```python
from build123d import *

# Parameters (mm, degrees)
ESBO_O1_W                = 50
ESBO_O1_H                = 11
RESSALTO_EXTRUS_O1_DEPTH = 22.5
ESBO_O2_W                = 46
ESBO_O2_H                = 7
CORTE_EXTRUS_O1_DEPTH    = 20.5
ESBO_O3_W                = 10.97916057
ESBO_O3_H                = 2
CORTE_EXTRUS_O2_DEPTH    = 4
CORTE_EXTRUS_O3_DEPTH    = 4
ESBO_O9_W                = 50
ESBO_O9_H                = 4
RESSALTO_EXTRUS_O4_DEPTH = 7
ESBO_O13_R               = 1.5
CORTE_EXTRUS_O4_DEPTH    = 7
ESBO_O19_W               = 9
ESBO_O19_H               = 4
RESSALTO_EXTRUS_O5_DEPTH = 22.5
ESBO_O20_R               = 1.7
RESSALTO_EXTRUS_O7_DEPTH = 3.5
ESBO_O21_W               = 68.510383691
ESBO_O21_H               = 66.833312069
CORTE_EXTRUS_O7_DEPTH    = 50.144843501
CORTE_EXTRUS_O8_DEPTH    = 35.762993058
RESSALTO_EXTRUS_O9_DEPTH = 3.5
ESBO_O24_R               = 1.6
CORTE_EXTRUS_O9_DEPTH    = 3.5


with BuildPart() as part:
    # Esboço1 → Ressalto-extrusão1 (new body)
    with BuildSketch(Plane(origin=(0, 0, 0), x_dir=(1, 0, 0), z_dir=(0, 1, 0))):
        Rectangle(ESBO_O1_W, ESBO_O1_H)
    extrude(amount=RESSALTO_EXTRUS_O1_DEPTH)

    # Esboço2 → Corte-extrusão1 (cut)
    with BuildSketch(Plane(origin=(0, 22.5, 0), x_dir=(1, 0, 0), z_dir=(0, 1, 0))):
        Rectangle(ESBO_O2_W, ESBO_O2_H)
    extrude(amount=-CORTE_EXTRUS_O1_DEPTH, mode=Mode.SUBTRACT)

    # Esboço3 → Corte-extrusão2 (cut)
    with BuildSketch(Plane(origin=(0, 22.5, 0), x_dir=(1, 0, 0), z_dir=(0, 1, 0))):
        with Locations((0, 4.5)):
            Rectangle(ESBO_O3_W, ESBO_O3_H)
    extrude(amount=-CORTE_EXTRUS_O2_DEPTH, mode=Mode.SUBTRACT)

    # Esboço5 → Corte-extrusão3 (cut)
    with BuildSketch(Plane.XY.offset(5.5)):
        with BuildLine():
            Line((-21, 22.5), (-4.5, 22.5))
            Line((-4.5, 22.5), (-4.5, 11.75))
            ThreePointArc((-4.5, 11.75), (-12.75, 3.5), (-21, 11.75))
            Line((-21, 11.75), (-21, 22.5))
        make_face()
        with BuildLine():
            Line((4.5, 22.5), (21, 22.5))
            Line((21, 22.5), (21, 11.75))
            ThreePointArc((21, 11.75), (12.75, 3.5), (4.5, 11.75))
            Line((4.5, 11.75), (4.5, 22.5))
        make_face()
    extrude(amount=-CORTE_EXTRUS_O3_DEPTH, mode=Mode.SUBTRACT)

    # Esboço9 → Ressalto-extrusão4 (add)
    with BuildSketch(Plane(origin=(0, 0, -5.5), x_dir=(-1, 0, 0), z_dir=(0, 0, -1))):
        with Locations((0, 2)):
            Rectangle(ESBO_O9_W, ESBO_O9_H)
    extrude(amount=RESSALTO_EXTRUS_O4_DEPTH)

    # Esboço13 → Corte-extrusão4 (cut)
    with BuildSketch(Plane(origin=(0, 4, 0), x_dir=(1, 0, 0), z_dir=(0, 1, 0))):
        with Locations(Location((10, 9, 0), (0, 0, 270))):
            Circle(ESBO_O13_R)
        with Locations(Location((5, 9, 0), (0, 0, 270))):
            Circle(ESBO_O13_R)
        with Locations(Location((20, 9, 0), (0, 0, 270))):
            Circle(ESBO_O13_R)
        with Locations(Location((15, 9, 0), (0, 0, 270))):
            Circle(ESBO_O13_R)
        with Locations(Location((0, 9, 0), (0, 0, 270))):
            Circle(ESBO_O13_R)
        with Locations(Location((-5, 9, 0), (0, 0, 270))):
            Circle(ESBO_O13_R)
        with Locations(Location((-10, 9, 0), (0, 0, 270))):
            Circle(ESBO_O13_R)
        with Locations(Location((-15, 9, 0), (0, 0, 270))):
            Circle(ESBO_O13_R)
        with Locations(Location((-20, 9, 0), (0, 0, 270))):
            Circle(ESBO_O13_R)
    extrude(amount=-CORTE_EXTRUS_O4_DEPTH, mode=Mode.SUBTRACT)

    # Esboço19 → Ressalto-extrusão5 (add)
    with BuildSketch(Plane(origin=(0, 22.5, 0), x_dir=(1, 0, 0), z_dir=(0, 1, 0))):
        with Locations((0, -5.5)):
            Rectangle(ESBO_O19_W, ESBO_O19_H)
    extrude(amount=-RESSALTO_EXTRUS_O5_DEPTH)

    # Esboço21 → Corte-extrusão7 (cut, through all)
    with BuildSketch(Plane(origin=(0, 32.5, 0), x_dir=(1, 0, 0), z_dir=(0, 1, 0))):
        with Locations((0.009195905, -3.607588671)):
            Rectangle(ESBO_O21_W, ESBO_O21_H)
    extrude(amount=-CORTE_EXTRUS_O7_DEPTH, mode=Mode.SUBTRACT)


with BuildPart() as body_2:
    # Esboço20 → Ressalto-extrusão7 (new body)
    with BuildSketch(Plane(origin=(0, 32.5, 0), x_dir=(1, 0, 0), z_dir=(0, 1, 0))):
        with BuildLine():
            ThreePointArc((8.833758049, 9), (15.166879024, 15.336707535), (21.5, 9))
            ThreePointArc((21.5, 9), (10.778241796, -16.658684905), (-15, -27.089718411))
            ThreePointArc((-15, -27.089718411), (-20.92850101, -21.097213824), (-15, -15.104709238))
            ThreePointArc((-15, -15.104709238), (1.873258871, -7.953021825), (8.833758049, 9))
        make_face()
        with Locations(Location((15, 9, 0), (0, 0, 270))):
            Circle(ESBO_O20_R, mode=Mode.SUBTRACT)
        with Locations(Location((-15, -21, 0), (0, 0, 270))):
            Circle(ESBO_O20_R, mode=Mode.SUBTRACT)
    extrude(amount=RESSALTO_EXTRUS_O7_DEPTH)

    # Esboço22 → Corte-extrusão8 (cut, through all)
    with BuildSketch(Plane(origin=(0, 36, 0), x_dir=(1, 0, 0), z_dir=(0, 1, 0))):
        with BuildLine():
            ThreePointArc((1.24551884, -16.20086225), (-1.05060257, -15.613093269), (-1.702635259, -17.891798883))
            ThreePointArc((-1.702635259, -17.891798883), (-0.204800523, -17.087752178), (1.24551884, -16.20086225))
        make_face()
        with BuildLine():
            ThreePointArc((1.24551884, -16.20086225), (-0.204800523, -17.087752178), (-1.702635259, -17.891798883))
            ThreePointArc((-1.702635259, -17.891798883), (0.209735934, -18.736436358), (1.495199477, -17.087752178))
            ThreePointArc((1.495199477, -17.087752178), (1.43158924, -16.627069487), (1.24551884, -16.20086225))
        make_face()
        with BuildLine():
            ThreePointArc((-5.840861487, -19.595514274), (-7.908251051, -18.436399829), (-9.12497893, -20.470415359))
            ThreePointArc((-9.12497893, -20.470415359), (-7.470627834, -20.079106718), (-5.840861487, -19.595514274))
        make_face()
        with BuildLine():
            ThreePointArc((-5.840861487, -19.595514274), (-7.470627834, -20.079106718), (-9.12497893, -20.470415359))
            ThreePointArc((-9.12497893, -20.470415359), (-7.273646696, -21.767655927), (-5.770627834, -20.079106718))
            ThreePointArc((-5.770627834, -20.079106718), (-5.788277872, -19.834773739), (-5.840861487, -19.595514274))
        make_face()
        with BuildLine():
            ThreePointArc((7.222954726, -11.091822097), (4.852915515, -11.115487395), (4.809999578, -13.485256187))
            ThreePointArc((4.809999578, -13.485256187), (6.050104938, -12.3224412), (7.222954726, -11.091822097))
        make_face()
        with BuildLine():
            ThreePointArc((7.222954726, -11.091822097), (6.050104938, -12.3224412), (4.809999578, -13.485256187))
            ThreePointArc((4.809999578, -13.485256187), (6.675333252, -13.903292096), (7.750104938, -12.3224412))
            ThreePointArc((7.750104938, -12.3224412), (7.612770072, -11.653055152), (7.222954726, -11.091822097))
        make_face()
        with BuildLine():
            ThreePointArc((11.686065273, -4.607737974), (9.402313913, -5.241871738), (9.972049301, -7.542534141))
            ThreePointArc((9.972049301, -7.542534141), (10.870291219, -6.099218009), (11.686065273, -4.607737974))
        make_face()
        with BuildLine():
            ThreePointArc((11.686065273, -4.607737974), (10.870291219, -6.099218009), (9.972049301, -7.542534141))
            ThreePointArc((9.972049301, -7.542534141), (11.695817941, -7.585322188), (12.570291219, -6.099218009))
            ThreePointArc((12.570291219, -6.099218009), (12.332620849, -5.232273919), (11.686065273, -4.607737974))
        make_face()
        with BuildLine():
            ThreePointArc((14.327996178, 2.818153576), (12.285471778, 1.615764297), (13.430014274, -0.459728025))
            ThreePointArc((13.430014274, -0.459728025), (13.925059514, 1.166596116), (14.327996178, 2.818153576))
        make_face()
        with BuildLine():
            ThreePointArc((14.327996178, 2.818153576), (13.925059514, 1.166596116), (13.430014274, -0.459728025))
            ThreePointArc((13.430014274, -0.459728025), (14.937092886, -0.199342556), (15.625059514, 1.166596116))
            ThreePointArc((15.625059514, 1.166596116), (15.262032275, 2.216597942), (14.327996178, 2.818153576))
        make_face()
    extrude(amount=-CORTE_EXTRUS_O8_DEPTH, mode=Mode.SUBTRACT)

    # Esboço23 → Ressalto-extrusão9 (add)
    with BuildSketch(Plane(origin=(0, 36, 0), x_dir=(1, 0, 0), z_dir=(0, 1, 0))):
        Polygon((15, 10.7), (23.5, 10.7), (23.5, 21), (6.5, 21), (6.5, 10.7), align=None)
    extrude(amount=-RESSALTO_EXTRUS_O9_DEPTH)

    # Esboço24 → Corte-extrusão9 (cut)
    with BuildSketch(Plane(origin=(0, 36, 0), x_dir=(1, 0, 0), z_dir=(0, 1, 0))):
        with Locations(Location((11.2, 15.85, 0), (0, 0, 270))):
            Circle(ESBO_O24_R)
        with Locations(Location((18.8, 15.85, 0), (0, 0, 270))):
            Circle(ESBO_O24_R)
    extrude(amount=-CORTE_EXTRUS_O9_DEPTH, mode=Mode.SUBTRACT)


solid = body_2.part
```
The model under review builds one solid part; all positions refer to its coordinate system, in mm. A direction names the side the tool comes from. Give positions to 0.01 mm unless a question says otherwise; leave off trailing zeros. Loops run counter-clockwise (first coordinate to the right, second up) from the corner with the lowest first, then second, coordinate; pieces in that order, holes last. Notation, with made-up numbers: (-32, 21) -> (-14, 21) arc R8 cw to (-14, 33) -> close; hole circle Ø5 at (-40, 72). An arc over 180 degrees is marked (long way). Use CSV: the item, a comma, the result in double quotes.
1. Consider section C-C, the plane z = -16. Write out the cut boundary in (x, y), then the cut area to 3 significant figures.
Result:
outline,"(6.5, 32.5) -> (9.61, 32.5) -> (9.61, 36) -> (6.5, 36) -> close; (12.79, 32.5) -> (17.21, 32.5) -> (17.21, 36) -> (12.79, 36) -> close; (20.39, 32.5) -> (23.5, 32.5) -> (23.5, 36) -> (20.39, 36) -> close"
area,"37.2 mm²"
2. Consider section B-B, the plane x = 15. Write out the cut boundary in (y, z).
Result:
outline,"(32.5, -21) -> (36, -21) -> (36, -10.7) -> (32.5, -10.7) -> close; (32.5, -7.3) -> (36, -7.3) -> (36, -2.48) -> (32.5, -2.48) -> close; (32.5, 0.15) -> (36, 0.15) -> (36, 11.65) -> (32.5, 11.65) -> close"
3. For P1, Ø2, axis at x = 1.5, y = 33.5, coming from the +Z side; P2, Ø1.3, axis at x = 8.5, y = 33.5, coming from the +Z side; P3, Ø2, axis at x = -7.5, y = 35.5, coming from the -Z side, all flat-tipped, find the tip position at first contact; note any pin that passes through.
Result:
P1,"stops at z = 23.78"
P2,"stops at z = 19.26"
P3,"stops at z = 13.46"
4. Machinability: for faces 1 (the face through (15, 34, -21)), 2 (the face through (6.5, 34, -16)), 3 (the face through (8, 34, -10.7)), which of the approach directions +Z, -Z, +X, -X, +Y, -Y give a long, thin tool a straight path to every point of the face, cutting with its end or side? Answer none if there is none.
Result:
face 1,"-Z, +X, -X, +Y, -Y"
face 2,"-Z, -X, +Y, -Y"
face 3,"-X, +Y, -Y"
5. Consider section A-A, the plane y = 34. Count the separate pieces of the cut face and the enclosed holes in it, then the cut area to 3 significant figures.
Result:
separate pieces,"1"
enclosed holes,"9"
area,"760 mm²"
6. Consider section D-D, the plane x = -6.5. Write out the cut boundary in (y, z).
Result:
outline,"(32.5, 13.46) -> (36, 13.46) -> (36, 18.68) -> (32.5, 18.68) -> close; (32.5, 21.47) -> (36, 21.47) -> (36, 26.17) -> (32.5, 26.17) -> close"
7. To check wall thickness, follow probe 1 along X at (y, z) = (34.4, -15.85); probe 2 along Z at (x, y) = (15, 34.5); probe 3 along Z at (x, y) = (12, 32.75). State the ranges of each line that lie inside material, in increasing order. Write a range as from..to.
Result:
probe 1,"x = 6.5..9.6, 12.8..17.2, 20.4..23.5"
probe 2,"z = -21..-10.7, -7.3..-2.48, 0.15..11.65"
probe 3,"z = -21..-17.24, -14.46..4.83, 7.37..15.39"
8. The part is to be moulded in two halves that separate along X. For faces 4 (the face through (-15.65, 34.23, 22.57)), 5 (the face through (6, 32.5, 3)), 6 (the face through (1.687, 34.226, 8.139)), say which applies: +X half, -X half, draft (parallel to the pull), parting line (faces both ways), or undercut.
Result:
face 4,"undercut"
face 5,"draft"
face 6,"-X half"
